from build123d import *

# Parameters (mm, degrees)
F0_R     = 31.5
F1_DEPTH = 20


with BuildPart() as f1:
    # F0 (on Top) → F1 (new body)
    with BuildSketch(Plane.XY):
        with BuildLine():
            ThreePointArc((-36.75, 0), (-39.0911135624, 6.9544805142), (-45.1612694301, 11.0774430022))
            ThreePointArc((-45.1612694301, 11.0774430022), (-45.5976101671, 9.1163560183), (-45.9488341969, 7.1382516029))
            ThreePointArc((-45.9488341969, 7.1382516029), (-42.1874616074, 4.4153854009), (-40.75, 0))
            ThreePointArc((-40.75, 0), (-42.1874616074, -4.4153854009), (-45.9488341969, -7.1382516029))
            ThreePointArc((-45.9488341969, -7.1382516029), (-45.5976101671, -9.1163560183), (-45.1612694301, -11.0774430022))
            ThreePointArc((-45.1612694301, -11.0774430022), (-39.0911135624, -6.9544805142), (-36.75, 0))
        make_face()
        with BuildLine():
            ThreePointArc((-45.1612694301, -11.0774430022), (5.579021935, -46.1641041747), (46.5, 0))
            ThreePointArc((46.5, 0), (5.579021935, 46.1641041747), (-45.1612694301, 11.0774430022))
            ThreePointArc((-45.1612694301, 11.0774430022), (-39.0911135624, 6.9544805142), (-36.75, 0))
            ThreePointArc((-36.75, 0), (-39.0911135624, -6.9544805142), (-45.1612694301, -11.0774430022))
        make_face()
        Circle(F0_R, mode=Mode.SUBTRACT)
    extrude(amount=F1_DEPTH)


solid = f1.part
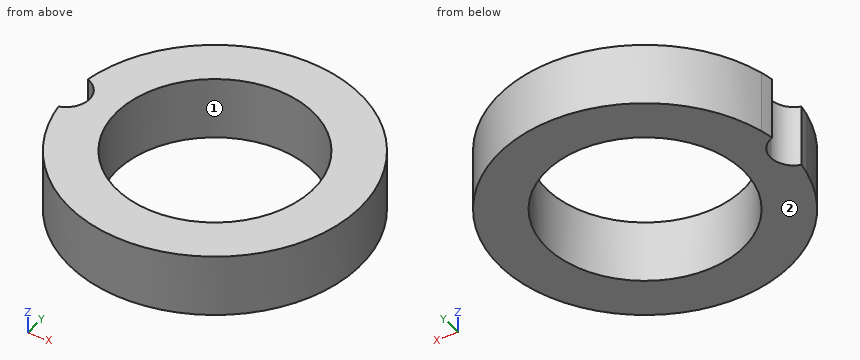
Can you work these out from the model? Positions are in its coordinate system, mm. Face numbers are marked on the shaded views. Round coordinates to 2 decimals unless told otherwise and drop trailing zeros. Order: outer loops, then holes, each group sorted by start corner. A loop starts at its lowest first (then second) coordinate and runs counter-clockwise, first axis right, second up. Notation, with made-up numbers: M 43,32.25 L 82,32.25 A28 ccw 82,58.25 Z; hole C -35.5,-36.5 d3. An arc over 180 degrees is marked long. Use a Markdown table: item, result.
1) Imagine slicing it at C-C (z = 3.75). List the corners of the cut face in (x, y) for me, then the cut area to 3 significant figures.
Geometry says:
| item | result |
|---|---|
| outline | M -45.95,-7.14 A46.5 ccw long -45.95,7.14 A7.5 cw Z; hole C 0,0 d63 |
| area | 3,620 mm² |
2) If I drill on line 1 along Y through (x, z) = (0, 14.25); line 2 along Y through (x, z) = (24.5, 5); line 3 along X through (y, z) = (25.5, 6.5), over which ranges is the centre line in solid material (lowest first)?
Geometry says:
| item | result |
|---|---|
| line 1 | y = -46.5 to -31.5, 31.5 to 46.5 |
| line 2 | y = -39.52 to -19.8, 19.8 to 39.52 |
| line 3 | x = -38.88 to -18.49, 18.49 to 38.88 |
3) Imagine slicing it at B-B (y = -26). List the corners of the cut face in (x, z) for me.
Geometry says:
| item | result |
|---|---|
| outline | M -38.55,0 L -17.78,0 L -17.78,20 L -38.55,20 Z; M 17.78,0 L 38.55,0 L 38.55,20 L 17.78,20 Z |
4) If we mould it in two halves opening along Y, with no side actions, what happens to the marked faces 1 and 2? For each: +Y half, -Y half, draft (parallel to the pull), parting line (faces both ways), or undercut.
Geometry says:
| item | result |
|---|---|
| face 1 | undercut |
| face 2 | draft |
5) Imagine slicing it at A-A (x = 0). List the corners of the cut face in (y, z) for me, then the cut area to 3 significant figures.
Geometry says:
| item | result |
|---|---|
| outline | M -46.5,0 L -31.5,0 L -31.5,20 L -46.5,20 Z; M 31.5,0 L 46.5,0 L 46.5,20 L 31.5,20 Z |
| area | 600 mm² |
6) I'm going to push flat-ended pins straight in: P1, Ø5, axis at y = 7.5, z = 4, coming from the -X side; P2, Ø1, axis at x = -10, z = 13, coming from the -Y side; P3, Ø1.5, axis at x = -14, z = 15.5, coming from the +Y side; P4, Ø4, axis at x = 25, z = 6, coming from the +Y side. Where does each tip first touch, or does it pass through?
Geometry says:
| item | result |
|---|---|
| P1 | stops at x = -45.95 |
| P2 | stops at y = -45.52 |
| P3 | stops at y = 44.57 |
| P4 | stops at y = 40.41 |
7) Imagine slicing it at D-D (y = -37). List the corners of the cut face in (x, z) for me, then the cut area to 3 significant figures.
Geometry says:
| item | result |
|---|---|
| outline | M -28.16,0 L 28.16,0 L 28.16,20 L -28.16,20 Z |
| area | 1,130 mm² |
